Part model, mm, in its own coordinate system. A direction names the side the tool comes from. Round coordinates to 2 decimals unless told otherwise and drop trailing zeros. Loops run counter-clockwise (first coordinate to the right, second up) from the corner with the lowest first, then second, coordinate; pieces in that order, holes last.
Autodesk Inventor part; units mm, degrees
ref_plane "YZ Plane" through (0, 0, 0) normal (1, 0, 0) x (0, 1, 0)
ref_plane "XZ Plane" through (0, 0, 0) normal (0, 1, 0) x (-1, 0, 0)
ref_plane "XY Plane" through (0, 0, 0) normal (0, 0, 1) x (1, 0, 0)
sketch "Sketch1" plane through (0, 0, 0) normal (0, 0, 1) x (1, 0, 0)
  line L0 (-3, 0) -> (-3, 20)
  line L1 (-15, 0) -> (-3, 0)
  line L2 (-15, 4) -> (-15, 0)
  line L3 (-7, 4) -> (-15, 4)
  line L4 (-7, 20) -> (-7, 4)
  line L5 (-3, 20) -> (-7, 20)
extrude "Extrusion4" add sketch "Sketch1" along normal blind 40
sketch "Sketch2" plane through (-15, 4, 0) normal (0, 1, 0) x (1, 0, 0)
  arc A0 (5.591, -13.591) -> (2.409, -13.591) centre (4, -12) ccw
  line L0 (4, -15.182) -> (5.591, -13.591)
  line L1 (2.409, -13.591) -> (4, -15.182)
  line L2 (8, 0) -> (0, 0)
  line L3 (0, 0) -> (0, -40)
  arc A1 (5.591, -29.591) -> (2.409, -29.591) centre (4, -28) ccw
  line L4 (4, -31.182) -> (5.591, -29.591)
  line L5 (2.409, -29.591) -> (4, -31.182)
  line L6 (8, -40) -> (0, -40)
  dimension "d8" = 2.25
  dimension "d9" = 12
  dimension "d10" = 4
  dimension "d11" = 2.25
  dimension "d12" = 2.25
  dimension "d13" = 2.25
  dimension "d14" = 12
  dimension "d15" = 4
extrude "Extrusion3" cut sketch "Sketch2" against normal blind 4
sketch "Sketch3" plane through (-7, 4, 0) normal (-1, 0, 0) x (0, 0, 1)
  arc A0 (7.091, 12.591) -> (7.091, 9.409) centre (5.5, 11) ccw
  line L0 (8.682, 11) -> (7.091, 9.409)
  line L1 (7.091, 12.591) -> (8.682, 11)
extrude "Extrusion2" cut sketch "Sketch3" against normal blind 4 draft 0
sketch "Sketch4" plane through (-7, 4, 0) normal (-1, 0, 0) x (0, 0, 1)
  arc A0 (36.091, 12.591) -> (36.091, 9.409) centre (34.5, 11) ccw
  line L0 (37.682, 11) -> (36.091, 9.409)
  line L1 (36.091, 12.591) -> (37.682, 11)
extrude "Extrusion1" cut sketch "Sketch4" against normal blind 4 draft 0
sketch "Sketch5" plane through (-3, 0, 0) normal (1, 0, 0) x (0, 0, -1)
  arc A0 (-36.091, 13.409) -> (-36.091, 16.591) centre (-34.5, 15) ccw
  line L0 (-40, 0) -> (-40, 20)
  circle A1 centre (-34.5, 15) radius 6.5 construction
  line L1 (0, 0) -> (-40, 0)
  line L2 (-37, 0) -> (-39.886, 8.1769)
  arc A2 (-40, 8.8426) -> (-39.886, 8.1769) centre (-38, 8.8426) ccw
  line L3 (-37, 0) -> (-40, 0)
  line L4 (-40, 0) -> (-40, 8.8426)
  line L5 (-20, 22.0768) -> (-20, -2.8383) construction
  line L6 (-3, 0) -> (-0.114, 8.1769)
  arc A3 (-0.114, 8.1769) -> (0, 8.8426) centre (-2, 8.8426) ccw
  line L7 (-3, 0) -> (0, 0)
  line L8 (0, 0) -> (0, 8.8426)
  point P0 (-40, 8.5)
  dimension "d16" = 13
  dimension "d17" = 3
  dimension "d18" = 6.5
  dimension "d19" = 2
extrude "Extrusion7" cut sketch "Sketch5" against normal through all
properties part number "Y-axis Belt Idler 1" material "ASA Plastic"
1) Slice it at D-D, the plane z = 25. Give the cut face in (x, y).
Values:
outline: (-15, 0) - (-3, 0) - (-3, 20) - (-7, 20) - (-7, 4) - (-15, 4) - close
2) Slice it at C-C, the plane y = 2.5. Give the cut face in (x, z).
Values:
outline: (-15, 2.12) - (-3, 2.12) - (-3, 37.88) - (-15, 37.88) - close; hole (-12.59, 13.59) arc R2.25 ccw (long way) to (-9.41, 13.59) - (-11, 15.18) - close; hole (-12.59, 29.59) arc R2.25 ccw (long way) to (-9.41, 29.59) - (-11, 31.18) - close
3) Mould opens along Z. For faces 1 (the face through (-5, 20, 20)), 2 (the face through (-5.028, 15.807, 7.875)), 3 (the face through (-7.58, 3.12, 1.9)), 4 (the face through (-7.58, 3.12, 38.1)) say: released by +Z, released by -Z, zero draft, split by the parting line, or undercut.
Values:
face 1: zero draft
face 2: undercut
face 3: released by -Z
face 4: released by +Z
4) Slice it at A-A, the plane z = 12. Give the cut face in (x, y).
Values:
outline: (-15, 0) - (-13.25, 0) - (-13.25, 4) - (-15, 4) - close; (-8.75, 0) - (-3, 0) - (-3, 20) - (-7, 20) - (-7, 4) - (-8.75, 4) - close
5) Slice it at B-B, the plane x = -5.5. Give the cut face in (y, z).
Values:
outline: (0, 3) - (8.18, 0.11) arc R2 ccw to (8.84, 0) - (20, 0) - (20, 40) - (8.84, 40) arc R2 ccw to (8.18, 39.89) - (0, 37) - close; hole (13.41, 7.09) arc R2.25 ccw (long way) to (16.59, 7.09) - (15, 8.68) - close; hole (13.41, 36.09) arc R2.25 ccw (long way) to (16.59, 36.09) - (15, 37.68) - close
6) Tool access for faces 5 (the face through (-11.807, 2.028, 14.375)), 6 (the face through (-9, 0, 20)), 7 (the face through (-5.03, 14.22, 36.9)), 8 (the face through (-11, 4, 20)), 9 (the face through (-3, 10, 20)): list every direction of +Z, -Z, +X, -X, +Y, -Y with a clear straight run to the whole face (end or side of a thin tool).
Values:
face 5: +Y, -Y
face 6: +Z, -Z, +X, -X, -Y
face 7: +X, -X
face 8: +Z, -Z, -X, +Y
face 9: +Z, -Z, +X, +Y, -Y
7) Drop flat-ended pins along their axis: pin 1 Ø4 at (x, z) = (-10, 23) entering from +Y; pin 2 Ø5 at (y, z) = (12.5, 33.5) entering from -X; pin 3 Ø4 at (y, z) = (15, 5.5) entering from -X. Give the stop position or say it passes through.
Values:
pin 1: stops at y = 4
pin 2: stops at x = -7
pin 3: passes through
8) Wall check: line 1 along X through (y, z) = (1.35, 28); line 2 along Z through (x, y) = (-10.75, 3); line 3 along X through (y, z) = (11.5, 34). Give the ranges that are in metal, low to high.
Values:
line 1: x = -15 to -13.25, -8.75 to -3
line 2: z = 1.94 to 9.76, 14.93 to 25.76, 30.93 to 38.06
line 3: x = -7 to -3
